Autodesk Inventor part; units mm, degrees
ref_plane "YZ Plane" through (0, 0, 0) normal (1, 0, 0) x (0, 1, 0)
ref_plane "XZ Plane" through (0, 0, 0) normal (0, 1, 0) x (-1, 0, 0)
ref_plane "XY Plane" through (0, 0, 0) normal (0, 0, 1) x (1, 0, 0)
sketch "Sketch1" plane through (0, 0, 0) normal (0, 1, 0) x (-1, 0, 0)
  circle A0 centre (0, 0) radius 10
  dimension "d0" = 20
extrude "Extrusion1" add sketch "Sketch1" along normal blind 15
fillet "Fillet1" radius 2.5 1 edges at (10, 15, 0)
sketch "Sketch2" plane through (0, 15, 0) normal (0, 1, 0) x (1, 0, 0)
  line L0 (-6.4787, 1.7612) -> (2.2441, 1.7612) construction
  line L1 (2.2441, 1.7612) -> (2.2441, -4.757) construction
  line L2 (2.2441, -4.757) -> (-6.4787, -4.757) construction
  line L3 (-6.4787, -4.757) -> (-6.4787, 1.7612) construction
  spline S0 degree 2 poles (-3.658, 0.1068) (-3.658, -0.3273) (-4.01, -1.0261) (-4.3054, -1.2213) knots 0 0 0 1 2 2 2
  spline S1 degree 2 poles (-4.3054, -1.2213) (-4.5469, -1.3729) (-5.0427, -1.4756) (-5.428, -1.4756) knots 0 0 0 1 2 2 2
  line L4 (-5.428, -1.4756) -> (-6.1576, -1.4756)
  line L5 (-6.1576, -1.4756) -> (-6.1576, 1.6944)
  line L6 (-6.1576, 1.6944) -> (-5.4357, 1.6944)
  spline S2 degree 2 poles (-5.4357, 1.6944) (-4.9887, 1.6944) (-4.4801, 1.5608) (-4.3003, 1.4426) knots 0 0 0 1 2 2 2
  spline S3 degree 2 poles (-4.3003, 1.4426) (-3.9946, 1.2397) (-3.658, 0.5692) (-3.658, 0.1068) knots 0 0 0 1 2 2 2
  spline S4 degree 2 poles (-4.0973, 0.112) (-4.0973, 0.4767) (-4.3388, 0.9931) (-4.5777, 1.1395) knots 0 0 0 1 2 2 2
  spline S5 degree 2 poles (-4.5777, 1.1395) (-4.7472, 1.2397) (-5.13, 1.3296) (-5.4152, 1.3296) knots 0 0 0 1 2 2 2
  line L7 (-5.4152, 1.3296) -> (-5.7363, 1.3296)
  line L8 (-5.7363, 1.3296) -> (-5.7363, -1.1108)
  line L9 (-5.7363, -1.1108) -> (-5.4152, -1.1108)
  spline S6 degree 2 poles (-5.4152, -1.1108) (-5.1351, -1.1108) (-4.7113, -1.0209) (-4.5392, -0.9002) knots 0 0 0 1 2 2 2
  spline S7 degree 2 poles (-4.5392, -0.9002) (-4.3182, -0.7512) (-4.0973, -0.258) (-4.0973, 0.112) knots 0 0 0 1 2 2 2
  spline S8 degree 2 poles (-0.9581, 1.3322) (-0.7783, 1.1215) (-0.5779, 0.505) (-0.5779, 0.1094) knots 0 0 0 1 2 2 2
  spline S9 degree 2 poles (-0.5779, 0.1094) (-0.5779, -0.276) (-0.7732, -0.9002) (-0.9581, -1.1108) knots 0 0 0 1 2 2 2
  spline S10 degree 2 poles (-0.9581, -1.1108) (-1.1534, -1.3318) (-1.6697, -1.5424) (-1.9806, -1.5424) knots 0 0 0 1 2 2 2
  spline S11 degree 2 poles (-1.9806, -1.5424) (-2.3017, -1.5424) (-2.8154, -1.3241) (-3.003, -1.1108) knots 0 0 0 1 2 2 2
  spline S12 degree 2 poles (-3.003, -1.1108) (-3.1854, -0.9002) (-3.3806, -0.2811) (-3.3806, 0.1094) knots 0 0 0 1 2 2 2
  spline S13 degree 2 poles (-3.3806, 0.1094) (-3.3806, 0.5076) (-3.1828, 1.1138) (-3.0004, 1.3322) knots 0 0 0 1 2 2 2
  spline S14 degree 2 poles (-3.0004, 1.3322) (-2.8154, 1.5428) (-2.2991, 1.7612) (-1.9806, 1.7612) knots 0 0 0 1 2 2 2
  spline S15 degree 2 poles (-1.9806, 1.7612) (-1.6569, 1.7612) (-1.138, 1.5351) (-0.9581, 1.3322) knots 0 0 0 1 2 2 2
  spline S16 degree 2 poles (-1.0172, 0.1094) (-1.0172, 0.4228) (-1.1534, 0.9083) (-1.2767, 1.0676) knots 0 0 0 1 2 2 2
  spline S17 degree 2 poles (-1.2767, 1.0676) (-1.4026, 1.232) (-1.7571, 1.3964) (-1.978, 1.3964) knots 0 0 0 1 2 2 2
  spline S18 degree 2 poles (-1.978, 1.3964) (-2.2066, 1.3964) (-2.5508, 1.2371) (-2.6819, 1.0676) knots 0 0 0 1 2 2 2
  spline S19 degree 2 poles (-2.6819, 1.0676) (-2.8077, 0.9057) (-2.9413, 0.4176) (-2.9413, 0.1094) knots 0 0 0 1 2 2 2
  spline S20 degree 2 poles (-2.9413, 0.1094) (-2.9413, -0.5149) (-2.4173, -1.1776) (-1.978, -1.1776) knots 0 0 0 1 2 2 2
  spline S21 degree 2 poles (-1.978, -1.1776) (-1.5387, -1.1776) (-1.0172, -0.5149) (-1.0172, 0.1094) knots 0 0 0 1 2 2 2
  line L10 (3.4372, 1.6944) -> (2.6409, -1.4756)
  line L11 (2.6409, -1.4756) -> (2.1682, -1.4756)
  line L12 (2.1682, -1.4756) -> (1.5234, 1.1549)
  line L13 (1.5234, 1.1549) -> (0.8966, -1.4756)
  line L14 (0.8966, -1.4756) -> (0.4291, -1.4756)
  line L15 (0.4291, -1.4756) -> (-0.3801, 1.6944)
  line L16 (-0.3801, 1.6944) -> (0.054, 1.6944)
  line L17 (0.054, 1.6944) -> (0.6911, -0.9336)
  line L18 (0.6911, -0.9336) -> (1.323, 1.6944)
  line L19 (1.323, 1.6944) -> (1.752, 1.6944)
  line L20 (1.752, 1.6944) -> (2.3891, -0.9644)
  line L21 (2.3891, -0.9644) -> (3.0236, 1.6944)
  line L22 (3.0236, 1.6944) -> (3.4372, 1.6944)
  line L23 (6.0832, -1.4756) -> (5.6105, -1.4756)
  line L24 (5.6105, -1.4756) -> (4.2079, 1.2577)
  line L25 (4.2079, 1.2577) -> (4.2079, -1.4756)
  line L26 (4.2079, -1.4756) -> (3.8148, -1.4756)
  line L27 (3.8148, -1.4756) -> (3.8148, 1.6944)
  line L28 (3.8148, 1.6944) -> (4.4134, 1.6944)
  line L29 (4.4134, 1.6944) -> (5.6901, -0.8154)
  line L30 (5.6901, -0.8154) -> (5.6901, 1.6944)
  line L31 (5.6901, 1.6944) -> (6.0832, 1.6944)
  line L32 (6.0832, 1.6944) -> (6.0832, -1.4756)
  point P0 (0, 0)
extrude "Extrusion2" cut sketch "Sketch2" against normal blind 5
sketch "Sketch3" plane through (0, 0, 0) normal (0, -1, 0) x (1, 0, 0)
  circle A0 centre (0, 0) radius 7.5
extrude "Extrusion3" cut sketch "Sketch3" against normal blind 2.5
properties part number "DOWN Button"
Work out the finished part from the listing and answer in its coordinate system (mm). A direction names the side the tool comes from. Coordinates: 2 decimals unless noted, no trailing zeros. Write each loop counter-clockwise with the first axis right and the second up, starting at its lowest first coordinate (ties: lowest second). Pieces come first, ordered by that corner, then holes.
Q1. Find the intervals of material crossed by line 1 (Z direction, x = 0, y = 0.55); line 2 (Y direction, x = -0.75, z = -2); line 3 (X direction, y = 3, z = -0.25), in increasing order.
Q2. Which of the six approach directions +Z, -Z, +X, -X, +Y, -Y give full straight-line access (tool end or side, diameter ignored) to faces 4 (the face through (4.208, 13, 0)), 5 (the face through (-2, 15, 0))?
Q3. Each of these flat-tipped pins is pushed along its axis until it touches: pin 1 Ø0.5 at (x, y) = (0.5, 12.5) entering from -Z; pin 2 Ø1.6 at (y, z) = (13.5, 0.5) entering from +X; pin 3 Ø4 at (y, z) = (11, -6) entering from +X. Where does it stop, or does it pass through?
Q4. A cutting plane is placed at A-A, the plane y = 6.75. Give the vertices of the cut face in (x, z), then the cut area to 3 significant figures.
Q5. Determine the mould class of faces 1 (the face through (2.17, 6.16, 9.76)), 2 (the face through (-4, 0, 7)), 3 (the face through (3.045, 12.535, -0.132)) for opening direction Z: released by +Z, released by -Z, zero draft, split by the parting line, or undercut.
Findings below:
1. line 1: z = -10 to -7.5, 7.5 to 10
1. line 2: y = 2.5 to 15
1. line 3: x = -10 to 10
2. face 4: +Y
2. face 5: +Z, -Z, +X, -X, +Y
3. pin 1: stops at z = -10
3. pin 2: stops at x = 9.99
3. pin 3: stops at x = 9.17
4. outline: circle Ø20 at (0, 0)
4. area: 314 mm2
5. face 1: split by the parting line
5. face 2: zero draft
5. face 3: undercut
